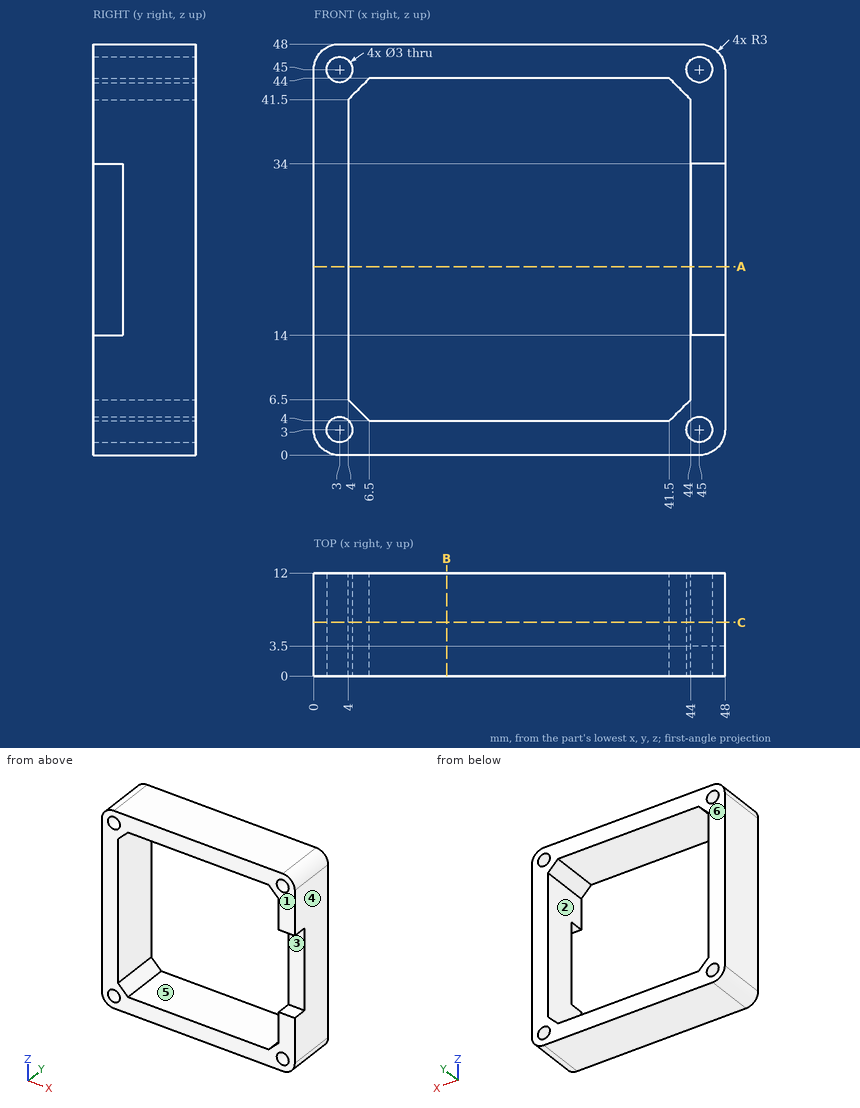
The figure shows three views and two pictorial views of one solid part (mm, origin at its lowest corner). Answer the questions. A direction names the side the tool comes from. Give positions to 0.01 mm unless a question says otherwise; leave off trailing zeros. Write each loop counter-clockwise with the first axis right and the second up, starting at its lowest first coordinate (ties: lowest second). Pieces come first, ordered by that corner, then holes. Notation, with made-up numbers: M -17,-23.75 L 24,-23.75 A20 ccw 24,9.25 Z; hole C 69.25,66.5 d10. An arc over 180 degrees is marked long. Write each question's results on one line, items separated by ' | '.
Q1. Consider L1, parallel to X at y = 8.75, z = 3; L2, parallel to Z at x = 36.5, y = 5.5. Determine where each line is inside the solid, lowest interval first. Write a range as from..to.
Output values:
L1: 0..1.5, 4.5..43.5, 46.5..48 | L2: 0..4, 44..48
Q2. Section C-C, the plane y = 6.25 is taken. Write down the section's boundary in (x, z), then the cut area to 4 significant figures.
Output values:
outline: M 0,3 A3 ccw 3,0 L 45,0 A3 ccw 48,3 L 48,45 A3 ccw 45,48 L 3,48 A3 ccw 0,45 Z; hole C 3,3 d3; hole C 3,45 d3; hole M 4,6.5 L 6.5,4 L 41.5,4 L 44,6.5 L 44,41.5 L 41.5,44 L 6.5,44 L 4,41.5 Z; hole C 45,3 d3; hole C 45,45 d3 | area: 680.5 mm2
Q3. For a pull along X with two mould halves and no side action, classify the marked faces 4, 5 and 6 as released by +X, released by -X, zero draft, split by the parting line, or undercut.
Output values:
face 4: released by +X | face 5: undercut | face 6: zero draft
Q4. Flat-ended cylindrical pins translate along their axes: P1, Ø2.5, axis at x = 45, z = 45, coming from the -Y side; P2, Ø3, axis at x = 46, z = 25.5, coming from the -Y side. Find the tip coordinate at first contact, or state that the pin passes through.
Output values:
P1: through | P2: y = 3.5
Q5. Section B-B, the plane x = 15.5 is taken. Write down the section's boundary in (y, z).
Output values:
outline: M 0,0 L 12,0 L 12,4 L 0,4 Z; M 0,44 L 12,44 L 12,48 L 0,48 Z
Q6. Section A-A, the plane z = 22 is taken. Write down the section's boundary in (x, y), then the cut area to 3 significant figures.
Output values:
outline: M 0,0 L 4,0 L 4,12 L 0,12 Z; M 44,3.5 L 48,3.5 L 48,12 L 44,12 Z | area: 82.0 mm2
Q7. A tool of negligible diameter and unlimited length cuts with its end or side. For the marked faces 1, 2 and 3, from which of +Z, -Z, +X, -X, +Y, -Y can it reach the whole face along a straight path? Write none if from no direction.
Output values:
face 1: +Z, -Z, +X, -X, -Y | face 2: +Y, -Y | face 3: +X, -Y
